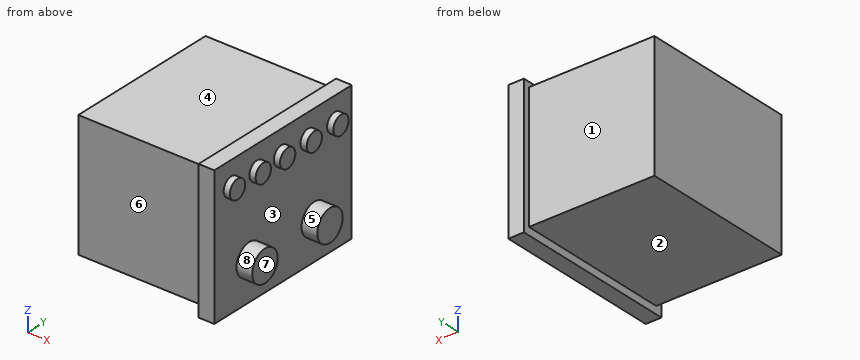
Autodesk Inventor part; units mm, degrees
ref_plane "YZ Plane" through (0, 0, 0) normal (1, 0, 0) x (0, 1, 0)
ref_plane "XZ Plane" through (0, 0, 0) normal (0, 1, 0) x (-1, 0, 0)
ref_plane "XY Plane" through (0, 0, 0) normal (0, 0, 1) x (1, 0, 0)
sketch "Sketch1" plane through (0, 0, 0) normal (1, 0, 0) x (0, 1, 0)
  line L0 (0, 0) -> (-63.5, 0)
  line L1 (-63.5, 0) -> (-63.5, -50.8)
  line L2 (-63.5, -50.8) -> (0, -50.8)
  line L3 (0, -50.8) -> (0, 0)
  dimension "d0" = 63.5
  dimension "d1" = 50.8
extrude "Extrusion1" add sketch "Sketch1" along normal blind 50.8
sketch "Sketch2" plane through (50.8, 0, 0) normal (1, 0, 0) x (0, 0, -1)
  line L0 (53.8638, 2.4661) -> (-2.0162, 2.4661)
  line L1 (-2.0162, 2.4661) -> (-2.0162, -66.1139)
  line L2 (-2.0162, -66.1139) -> (53.8638, -66.1139)
  line L3 (53.8638, -66.1139) -> (53.8638, 2.4661)
  point P0 (0, 0)
  dimension "d4" = 55.88
  dimension "d5" = 68.58
extrude "Extrusion2" add sketch "Sketch2" along normal blind 6.35
sketch "Sketch3" plane through (57.15, 0, 0) normal (1, 0, 0) x (0, 0, -1)
  circle A0 centre (38.2887, -16.224) radius 6.35
  circle A1 centre (38.2887, -48.6721) radius 6.35
  circle A2 centre (6.879, -6.1002) radius 3.81
  circle A3 centre (6.879, -18.8199) radius 3.81
  circle A4 centre (6.879, -34.395) radius 3.81
  circle A5 centre (6.879, -46.5954) radius 3.81
  circle A6 centre (6.879, -58.7959) radius 3.81
  point P0 (0, 0)
  dimension "d8" = 12.7
  dimension "d9" = 12.7
  dimension "d10" = 7.62
  dimension "d11" = 7.62
  dimension "d12" = 7.62
  dimension "d13" = 7.62
  dimension "d14" = 7.62
extrude "Extrusion3" add sketch "Sketch3" along normal blind 6.35 contours A0 | A1
sketch "Sketch4" plane through (57.15, 0, 0) normal (1, 0, 0) x (0, 0, -1)
  circle A0 centre (7.7755, -6.0244) radius 3.81
  circle A1 centre (7.7755, -19.3217) radius 3.81
  circle A2 centre (7.7755, -32.619) radius 3.81
  circle A3 centre (7.7755, -44.7893) radius 3.81
  circle A4 centre (7.7755, -57.6359) radius 3.81
  point P0 (0, 0)
  dimension "d17" = 7.62
  dimension "d18" = 7.62
  dimension "d19" = 7.62
  dimension "d20" = 7.62
  dimension "d21" = 7.62
extrude "Extrusion4" add sketch "Sketch4" along normal blind 2.54
sketch "Sketch5" plane through (57.15, 0, 0) normal (1, 0, 0) x (0, 0, -1)
  point P0 (0, 0)
sketch "Sketch6" plane through (57.15, 0, 0) normal (1, 0, 0) x (0, 0, -1)
  circle A0 centre (38.3083, -15.968) radius 3.175
  circle A1 centre (38.3083, -48.6538) radius 3.175
  point P0 (0, 0)
  dimension "d24" = 6.35
  dimension "d25" = 6.35
properties part number "Battery 2"
The model under review builds one solid part; all positions refer to its coordinate system, in mm. Face numbers are marked on the shaded views. A direction names the side the tool comes from. Round coordinates to 2 decimals unless told otherwise and drop trailing zeros. Loops run counter-clockwise (first coordinate to the right, second up) from the corner with the lowest first, then second, coordinate; pieces in that order, holes last. Notation, with made-up numbers: (9, -33.5) - (34, -33.5) arc R21 ccw to (34, -18.5) - close; hole circle Ø7 at (-25.5, -11.5). An arc over 180 degrees is marked (long way). Use a Markdown table: item, result. Add a question column.
Q1. Add section C-C (x = 31.5). State the section outline as (y, z) points, plus the area to 3 significant figures.
Q2. Add section A-A (y = -24.5). State the section outline as (x, z) points, plus the area to 3 significant figures.
Q3. The part is to be moulded in two halves that separate along Y. For the marked faces 5, 6, 7 and 8, say which applies: pulls with the +Y half, pulls with the -Y half, needs draft (parallel to the pull), parting line crosses it, or undercut.
Q4. Insertion check: pin 1 Ø8.5 at (y, z) = (-32.5, -6.5) entering from +X; pin 2 Ø1.5 at (x, z) = (32, -5) entering from -Y; pin 3 Ø4 at (y, z) = (-25, -6.5) entering from -X; pin 4 Ø1 at (x, y) = (50, -33) entering from -Z. Each pin has a flat end and moves straight along its axis. Give the tip position at first contact, or say it passes through.
Q5. Add section D-D (y = -11). State the section outline as (x, z) points.
Q6. Add section B-B (z = -9). State the section outline as (x, y) points.
Q7. For probe 1 along Y at (x, z) = (9, -49); probe 2 along Z at (x, y) = (41.5, -13.5); probe 3 along X at (y, z) = (-61, -27.5), list the stretches that pass through material, from the lowest coordinate up.
Q8. Machinability: for the marked faces 1, 2, 3 and 4, which of the approach directions +Z, -Z, +X, -X, +Y, -Y give a long, thin tool a straight path to every point of the face, cutting with its end or side? Answer none if there is none.
Worked answers:
| question | item | result |
|---|---|---|
| 1 | outline | (-63.5, -50.8) - (0, -50.8) - (0, 0) - (-63.5, 0) - close |
| 1 | area | 3,230 mm² |
| 2 | outline | (0, -50.8) - (50.8, -50.8) - (50.8, -53.86) - (57.15, -53.86) - (57.15, 2.02) - (50.8, 2.02) - (50.8, 0) - (0, 0) - close |
| 2 | area | 2,940 mm² |
| 3 | face 5 | undercut |
| 3 | face 6 | pulls with the -Y half |
| 3 | face 7 | needs draft |
| 3 | face 8 | undercut |
| 4 | pin 1 | x = 59.69 |
| 4 | pin 2 | y = -63.5 |
| 4 | pin 3 | x = 0 |
| 4 | pin 4 | z = -50.8 |
| 5 | outline | (0, -50.8) - (50.8, -50.8) - (50.8, -53.86) - (57.15, -53.86) - (57.15, -41.9) - (63.5, -41.9) - (63.5, -34.68) - (57.15, -34.68) - (57.15, 2.02) - (50.8, 2.02) - (50.8, 0) - (0, 0) - close |
| 6 | outline | (0, -63.5) - (50.8, -63.5) - (50.8, -66.11) - (57.15, -66.11) - (57.15, -61.24) - (59.69, -61.24) - (59.69, -54.03) - (57.15, -54.03) - (57.15, -48.4) - (59.69, -48.4) - (59.69, -41.18) - (57.15, -41.18) - (57.15, -36.23) - (59.69, -36.23) - (59.69, -29.01) - (57.15, -29.01) - (57.15, -22.93) - (59.69, -22.93) - (59.69, -15.71) - (57.15, -15.71) - (57.15, -9.63) - (59.69, -9.63) - (59.69, -2.42) - (57.15, -2.42) - (57.15, 2.47) - (50.8, 2.47) - (50.8, 0) - (0, 0) - close |
| 7 | probe 1 | -63.5 to 0 |
| 7 | probe 2 | -50.8 to 0 |
| 7 | probe 3 | 0 to 57.15 |
| 8 | face 1 | +Z, -Z, -X, +Y |
| 8 | face 2 | -Z, -X, +Y, -Y |
| 8 | face 3 | +X |
| 8 | face 4 | +Z, -X, +Y, -Y |
